```python
from build123d import *

# Parameters (mm, degrees)
SKETCH1_R           = 1
BOSS_EXTRUDE1_DEPTH = 2
SKETCH2_R           = 0.5
CUT_EXTRUDE1_DEPTH  = 0.5
SKETCH3_R           = 0.5
CUT_EXTRUDE2_DEPTH  = 0.5


with BuildPart() as part:
    # Sketch1 → Boss-Extrude1 (new body)
    with BuildSketch(Plane.XY):
        with BuildLine():
            Line((-19.041986571, 4), (19.041986571, 4))
            ThreePointArc((19.041986571, 4), (23.041986571, 0), (19.041986571, -4))
            Line((19.041986571, -4), (-19.041986571, -4))
            ThreePointArc((-19.041986571, -4), (-23.041986571, 0), (-19.041986571, 4))
        make_face()
        Circle(SKETCH1_R, mode=Mode.SUBTRACT)
        with Locations((19.041986571, 0)):
            Circle(SKETCH1_R, mode=Mode.SUBTRACT)
        with Locations((-19.041986571, 0)):
            Circle(SKETCH1_R, mode=Mode.SUBTRACT)
    extrude(amount=BOSS_EXTRUDE1_DEPTH)

    # Sketch2 → Cut-Extrude1 (cut)
    with BuildSketch(Plane(origin=(0, 4, 0), x_dir=(1, 0, 0), z_dir=(0, 1, 0))):
        with Locations((-19.041986571, -1)):
            Circle(SKETCH2_R)
        with Locations((19.041986571, -1)):
            Circle(SKETCH2_R)
    extrude(amount=-CUT_EXTRUDE1_DEPTH, mode=Mode.SUBTRACT)

    # Sketch3 → Cut-Extrude2 (cut)
    with BuildSketch(Plane.XZ.offset(4)):
        with Locations((0, 1)):
            Circle(SKETCH3_R)
    extrude(amount=-CUT_EXTRUDE2_DEPTH, mode=Mode.SUBTRACT)


solid = part.part
```
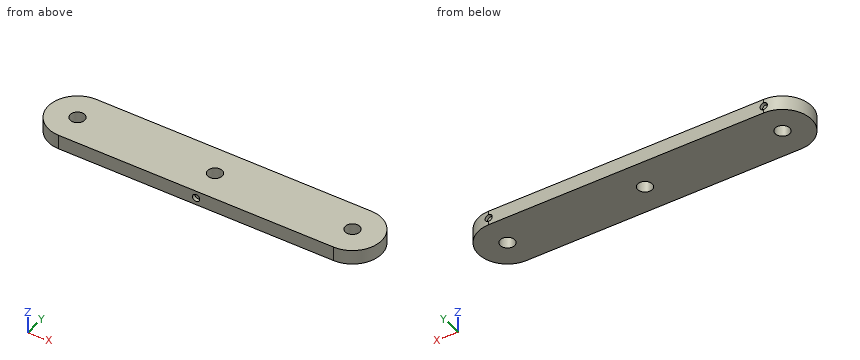
The listing builds one solid part. Answer for the finished solid, in the listing's coordinates (mm). Give positions to 0.01 mm unless a question says otherwise; leave off trailing zeros. Order: outer loops, then holes, each group sorted by start corner. A loop starts at its lowest first (then second) coordinate and runs counter-clockwise, first axis right, second up. Notation, with made-up numbers: (26.25, 77.25) -> (78.25, 77.25) arc R19 ccw to (78.25, 104.25) -> close; hole circle Ø10 at (23.25, 37). An arc over 180 degrees is marked (long way). Write each question's results on one line, items separated by ' | '.
Q1. Straight lines are drawn through the part: probe 1 along Y at (x, z) = (0, 1.2); probe 2 along X at (y, z) = (0.5, 1.6); probe 3 along Y at (x, z) = (19, 0.7). For each, find the intervals that lie inside material, in ascending order. Write a range as from..to.
Checked values:
probe 1: y = -3.5..-1, 1..4 | probe 2: x = -23.01..-19.91, -18.18..-0.87, 0.87..18.18, 19.91..23.01 | probe 3: y = -4..-1, 1..3.5
Q2. The part is cut by section C-C, the plane y = 2.25. Give the vertices of the cut face in (x, z).
Checked values:
outline: (-22.35, 0) -> (22.35, 0) -> (22.35, 2) -> (-22.35, 2) -> close
Q3. The part is cut by section A-A, the plane x = 0. Give the vertices of the cut face in (y, z), and give its area (3 significant figures).
Checked values:
outline: (-4, 0) -> (-1, 0) -> (-1, 2) -> (-4, 2) -> (-4, 1.5) -> (-3.5, 1.5) -> (-3.5, 0.5) -> (-4, 0.5) -> close; (1, 0) -> (4, 0) -> (4, 2) -> (1, 2) -> close | area: 11.5 mm^2
Q4. Each of these flat-tipped pins is pushed along its axis until it touches: P1, Ø3, axis at x = 19.04, y = 0, coming from the +Z side; P2, Ø1, axis at y = 3, z = 1, coming from the +X side; P3, Ø0.8, axis at x = 19, z = 1, coming from the +Y side. Where does it stop, or does it pass through?
Checked values:
P1: stops at z = 2 | P2: stops at x = 22.16 | P3: stops at y = 3.5
Q5. The part is cut by section D-D, the plane y = -3. Give the vertices of the cut face in (x, z), and give its area (3 significant figures).
Checked values:
outline: (-21.69, 0) -> (21.69, 0) -> (21.69, 2) -> (-21.69, 2) -> close | area: 86.8 mm^2
Q6. The part is cut by section B-B, the plane z = 1. Give the vertices of the cut face in (x, y).
Checked values:
outline: (-19.54, 3.5) -> (-19.54, 3.97) arc R4 ccw to (-19.04, -4) -> (-0.5, -4) -> (-0.5, -3.5) -> (0.5, -3.5) -> (0.5, -4) -> (19.04, -4) arc R4 ccw to (19.54, 3.97) -> (19.54, 3.5) -> (18.54, 3.5) -> (18.54, 4) -> (-18.54, 4) -> (-18.54, 3.5) -> close; hole circle Ø2 at (-19.04, 0); hole circle Ø2 at (0, 0); hole circle Ø2 at (19.04, 0)
